Could you check a few things on this drawing? It's one solid part, dimensions in mm from its lowest x, y, z. A direction names the side the tool comes from. Give positions to 0.01 mm unless a question says otherwise; leave off trailing zeros. Order: outer loops, then holes, each group sorted by start corner. A loop starts at its lowest first (then second) coordinate and runs counter-clockwise, first axis right, second up. Notation, with made-up numbers: M 81.25,55 L 112.25,55 A23 cw 112.25,71 Z; hole C 26,-11 d1. An arc over 180 degrees is marked long. Use one line per item in the form item = value.
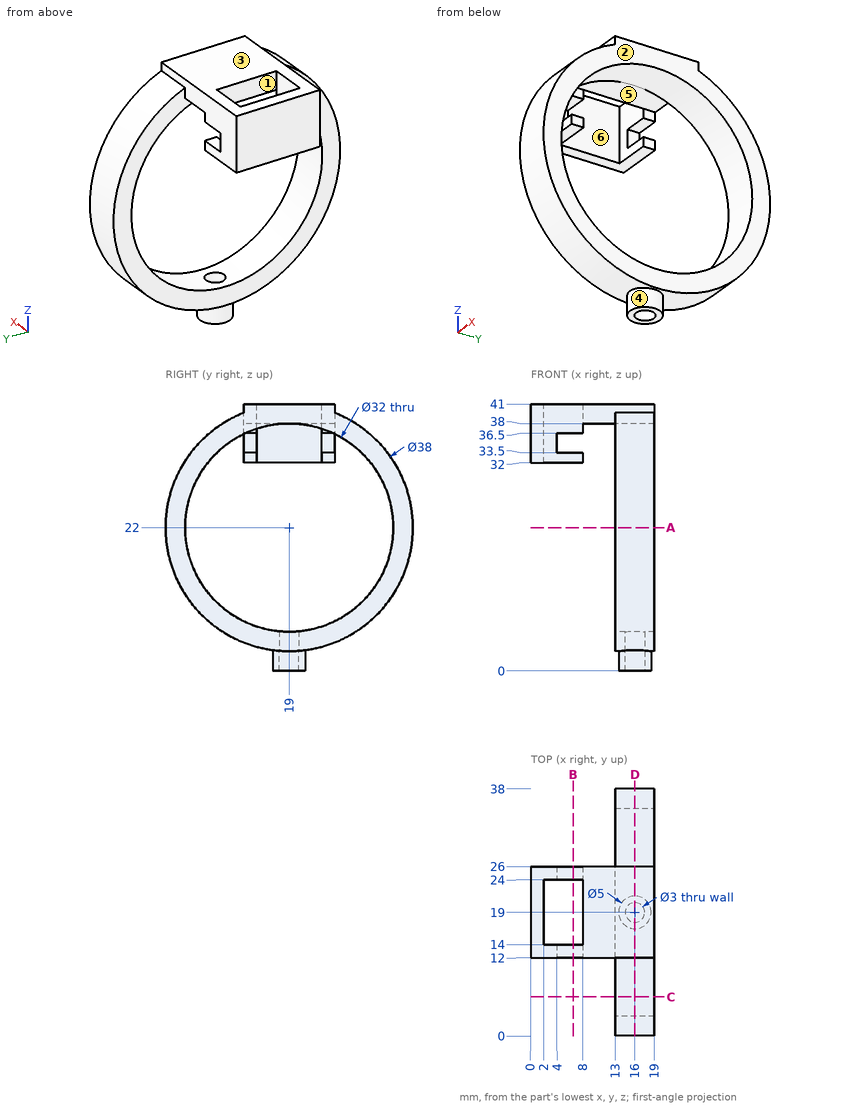
Q1. I want a section at B-B on x = 6.5. Write out the boundary of the cut face in (y, z), then the cut area to 3 significant figures.
Found:
outline = M 12,32 L 14,32 L 14,33.5 L 12,33.5 Z; M 12,36.5 L 14,36.5 L 14,41 L 12,41 Z; M 24,32 L 26,32 L 26,33.5 L 24,33.5 Z; M 24,36.5 L 26,36.5 L 26,41 L 24,41 Z
area = 24.0 mm²
Q2. I need wall thicknesses on L1, parallel to Y at x = 16, z = 1.7; L2, parallel to Z at x = 11.5, y = 12.5; L3, parallel to X at y = 21, z = 37.5. Which ranges of each line are inside material? Lowest first, please.
Found:
L1 = 16.5 to 17.5, 20.5 to 21.5
L2 = 38 to 41
L3 = 0 to 2
Q3. I'm going to push flat-ended pins straight in: pin 1 Ø10 at (y, z) = (17, 36.5) entering from -X; pin 2 Ø5 at (x, z) = (5.5, 35) entering from -Y; pin 3 Ø2.5 at (x, y) = (11, 16.5) entering from -Z; pin 4 Ø2 at (y, z) = (24.5, 35) entering from +X. Where does each tip first touch, or does it pass through?
Found:
pin_1 = 0
pin_2 = 12
pin_3 = 38
pin_4 = 4
Q4. Thinking about a two-plate mould opening in X: for the marked faces 1, 2 and 3, which applies, +X half, -X half, draft (parallel to the pull), parting line (faces both ways), or undercut?
Found:
face_1 = undercut
face_2 = +X half
face_3 = draft
Q5. I want a section at D-D on x = 16. Write out the boundary of the cut face in (y, z), then the cut area to 3 significant figures.
Found:
outline = M 12,39.66 A19 ccw 16.5,3.17 L 16.5,0 L 17.5,0 L 17.5,6.07 A16 cw long 20.5,6.07 L 20.5,0 L 21.5,0 L 21.5,3.17 A19 ccw 26,39.66 L 26,41 L 12,41 Z
area = 333 mm²
Q6. I want a section at C-C on y = 6. Write out the boundary of the cut face in (x, z).
Found:
outline = M 13,8.14 L 19,8.14 L 19,12.67 L 13,12.67 Z; M 13,31.33 L 19,31.33 L 19,35.86 L 13,35.86 Z
Q7. I want a section at A-A on z = 22. Write out the boundary of the cut face in (x, y), then the cut area to 3 significant figures.
Found:
outline = M 13,0 L 19,0 L 19,3 L 13,3 Z; M 13,35 L 19,35 L 19,38 L 13,38 Z
area = 36.0 mm²
Q8. On a 3-axis mill with a long thin cutter (end or side, diameter ignored), from which of +Z, -Z, +X, -X, +Y, -Y can I reach the whole of each face in a straight line? I mean the marked faces 4, 5 and 6. Say none if no direction works.
Found:
face_4 = -Z
face_5 = -Z, +Y, -Y
face_6 = +Z, -Z
